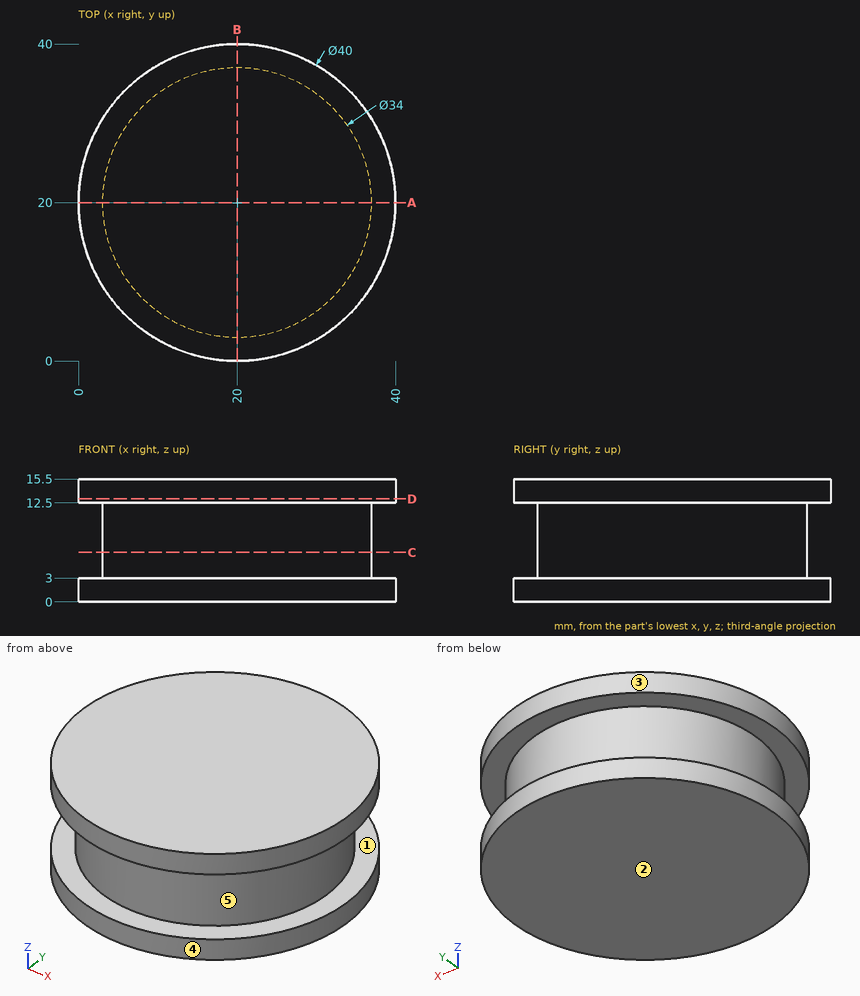
The drawing under review shows one solid part. Ordinate dimensions are in mm from its lowest x, y, z. A direction names the side the tool comes from. Round coordinates to 2 decimals unless told otherwise and drop trailing zeros. Write each loop counter-clockwise with the first axis right and the second up, starting at its lowest first coordinate (ties: lowest second). Pieces come first, ordered by that corner, then holes.
(1) We need section A-A on y = 20. Give the boundary of the cut face in (x, z).
(2) Mouldability with a two-part tool opening along Z and no side actions: class the marked faces 1, 2 and 3 as +Z half, -Z half, draft (parallel to the pull), parting line (faces both ways), or undercut.
(3) We need section D-D on z = 13. Give the boundary of the cut face in (x, y), and give its area (3 significant figures).
(4) Machinability: for the marked faces 4 and 5, which of the approach directions +Z, -Z, +X, -X, +Y, -Y give a long, thin tool a straight path to every point of the face, cutting with its end or side? Answer none if there is none.
(5) Wall thickness on L1, parallel to Z at x = 23, y = 3; L2, parallel to X at y = 20.5, z = 5.5; L3, parallel to X at y = 24.5, z = 14: over which ranges is each line inside the solid? List them lowest first.
(6) Insertion check: pin 1 (20 mm diameter, centred on x = 22.5, y = 27, fed in from -Z); pin 2 (1.5 mm diameter, centred on x = 21.5, z = 12.5, fed in from +Y); pin 3 (5 mm diameter, centred on x = 9, z = 5, fed in from -Y); pin 4 (2 mm diameter, centred on y = 13.5, z = 7.5, fed in from -X). Each pin has a flat end and moves straight along its axis. Give the tip position at first contact, or say it passes through.
(7) We need section C-C on z = 6.25. Give the boundary of the cut face in (x, y).
Findings below:
1. outline: (0, 0) - (40, 0) - (40, 3) - (37, 3) - (37, 12.5) - (40, 12.5) - (40, 15.5) - (0, 15.5) - (0, 12.5) - (3, 12.5) - (3, 3) - (0, 3) - close
2. face 1: undercut
2. face 2: -Z half
2. face 3: draft
3. outline: circle Ø40 at (20, 20)
3. area: 1,260 mm2
4. face 4: +Z, -Z
4. face 5: none
5. L1: z = 0 to 3, 12.5 to 15.5
5. L2: x = 3.01 to 36.99
5. L3: x = 0.51 to 39.49
6. pin 1: stops at z = 0
6. pin 2: stops at y = 39.99
6. pin 3: stops at y = 2.4
6. pin 4: stops at x = 3.91
7. outline: circle Ø34 at (20, 20)
